Autodesk Inventor part; units mm, degrees
ref_plane "YZ Plane" through (0, 0, 0) normal (1, 0, 0) x (0, 1, 0)
ref_plane "XZ Plane" through (0, 0, 0) normal (0, 1, 0) x (-1, 0, 0)
ref_plane "XY Plane" through (0, 0, 0) normal (0, 0, 1) x (1, 0, 0)
ref_plane "Work Plane1" through (0, 0, 0) normal (0, 0, 1) x (1, 0, 0)
sketch "Sketch1" plane through (0, 0, 0) normal (0, 0, 1) x (1, 0, 0)
  circle A0 centre (-10, -25) radius 1.45
  circle A1 centre (-10, 25) radius 1.45
  circle A2 centre (10, 25) radius 1.45
  circle A3 centre (10, -25) radius 1.45
  circle A4 centre (-25, 25) radius 2.325
  circle A5 centre (25, -25) radius 2.325
  circle A6 centre (-25, -25) radius 2.325
  circle A7 centre (25, 25) radius 2.325
  line L0 (28, 30) -> (30, 28)
  line L1 (28, 30) -> (-28, 30)
  line L2 (-30, 28) -> (-28, 30)
  line L3 (-30, 28) -> (-30, -28)
  line L4 (-28, -30) -> (-30, -28)
  line L5 (-28, -30) -> (28, -30)
  line L6 (30, -28) -> (28, -30)
  line L7 (30, -28) -> (30, 28)
  circle A8 centre (-17.5, -17.5) radius 1.95
  circle A9 centre (17.5, 17.5) radius 1.95
  circle A10 centre (17.5, -17.5) radius 1.95
  circle A11 centre (-17.5, 17.5) radius 1.95
  circle A12 centre (0, 0) radius 7.5
  circle A13 centre (-25.33, -75.26) radius 6.15
  circle A14 centre (25, -10) radius 1.45
  circle A15 centre (-25, -10) radius 1.45
  circle A16 centre (-25, 10) radius 1.45
  circle A17 centre (25, 10) radius 1.45
  point P0 (0, 0)
extrude "Extrusion1" add sketch "Sketch1" along normal blind 8 contours L0 L7 L6 L5 L4 L3 L2 L1
sketch "Sketch2" plane through (0, 0, 8) normal (0, 0, 1) x (1, 0, 0)
  circle A0 centre (0, 0) radius 7.5
  circle A1 centre (25, 10) radius 1.45
  circle A2 centre (-25, 10) radius 1.45
  circle A3 centre (-25, -10) radius 1.45
  circle A4 centre (25, -10) radius 1.45
  circle A5 centre (10, -25) radius 1.45
  circle A6 centre (10, 25) radius 1.45
  circle A7 centre (-10, 25) radius 1.45
  circle A8 centre (-10, -25) radius 1.45
  line L0 (-28, -30) -> (28, -30)
  line L1 (28, -30) -> (30, -28)
  line L2 (30, -28) -> (30, 28)
  line L3 (30, 28) -> (28, 30)
  line L4 (28, 30) -> (-28, 30)
  line L5 (30, -28) -> (30, 28)
  line L6 (30, -30) -> (18, -30)
  line L7 (18, -30) -> (18, -80)
  line L8 (18, -80) -> (30, -80)
  line L9 (30, -80) -> (30, -30)
  line L10 (30, 28) -> (30, -28)
  line L11 (30, -30) -> (30, -28)
  line L12 (30, -28) -> (28, -30)
  line L13 (-28, 30) -> (-30, 28)
  line L14 (-30, 28) -> (-30, -28)
  line L15 (-30, -28) -> (-28, -30)
  line L16 (-30, -30) -> (-18, -30)
  line L17 (-18, -30) -> (-18, -80)
  line L18 (-18, -80) -> (-30, -80)
  line L19 (-30, -80) -> (-30, -30)
  line L20 (-30, -30) -> (-30, -28)
  line L21 (-30, -28) -> (-28, -30)
  line L22 (-28, -30) -> (-30, -30)
  line L23 (28, -30) -> (30, -28)
  line L24 (28, -30) -> (30, -30)
  line L25 (30, -30) -> (30, -28)
  line L26 (30, -28) -> (28, -30)
  circle A9 centre (-17.5, 17.5) radius 1.95
  circle A10 centre (-25, 25) radius 2.325
  circle A11 centre (25, 25) radius 2.325
  circle A12 centre (17.5, 17.5) radius 1.95
  circle A13 centre (17.5, -17.5) radius 1.95
  circle A14 centre (25, -25) radius 2.325
  circle A15 centre (-25, -25) radius 2.325
  point P0 (0, 0)
  point P1 (-24.2387, -104)
  dimension "d57" = 12
  dimension "d58" = 50
  dimension "d59" = 12
extrude "Extrusion2" add sketch "Sketch2" along normal blind 7
fillet "Fillet1" radius 4 6 edges at (30, -80, 11.5) (18, -80, 11.5) (-18, -80, 11.5) (-30, -80, 11.5) (-18, -30, 11.5) (18, -30, 11.5)
sketch "Sketch6" plane through (0, 0, 15) normal (0, 0, 1) x (1, 0, 0)
  line L0 (30, -76) -> (30, 28)
  line L1 (30, 28) -> (28, 30)
  line L2 (28, 30) -> (-28, 30)
  circle A0 centre (-1.1442, -37.6316) radius 2.45
  circle A1 centre (-1.1442, -37.6316) radius 1.45 construction
  line L3 (-14, -30) -> (14, -30)
  line L4 (18, -34) -> (18, -76)
  line L5 (22, -80) -> (26, -80)
  line L6 (-28, 30) -> (-30, 28)
  line L7 (-30, 28) -> (-30, -76)
  line L8 (-26, -80) -> (-22, -80)
  line L9 (-18, -76) -> (-18, -34)
  arc A2 (-30, -76) -> (-26, -80) centre (-26, -76) ccw
  arc A3 (-22, -80) -> (-18, -76) centre (-22, -76) ccw
  arc A4 (-14, -30) -> (-18, -34) centre (-14, -34) ccw
  arc A5 (18, -34) -> (14, -30) centre (14, -34) ccw
  arc A6 (18, -76) -> (22, -80) centre (22, -76) ccw
  arc A7 (26, -80) -> (30, -76) centre (26, -76) ccw
  point P0 (0, 0)
  dimension "d27" = 4.9
extrude "Extrusion6" cut sketch "Sketch6" against normal blind 4 contours A0
ref_plane "Work Plane2" through (-6, -91, 19) normal (1, 0, 0) x (0, 0, -1)
sketch "Sketch7" plane through (0, 0, 15) normal (0, 0, 1) x (1, 0, 0)
  circle A0 centre (10, -25) radius 1.45
  circle A1 centre (-10, -25) radius 1.45
  circle A2 centre (-25, -10) radius 1.45
  circle A3 centre (-25, 10) radius 1.45
  circle A4 centre (-10, 25) radius 1.45
  circle A5 centre (10, 25) radius 1.45
  circle A6 centre (25, 10) radius 1.45
  circle A7 centre (25, -10) radius 1.45
  circle A8 centre (-25, 25) radius 2.325
  circle A9 centre (25, 25) radius 2.325
  circle A10 centre (25, -25) radius 2.325
  circle A11 centre (-25, -25) radius 2.325
  point P0 (0, 0)
hole "Hole1" at (-25, -10, 15) at (-25, 10, 15) at (-10, 25, 15) at (10, 25, 15) at (25, 10, 15) at (25, -10, 15) at (10, -25, 15) at (-10, -25, 15) at (-25, 25, 15) at (-25, -25, 15) at (25, -25, 15) at (25, 25, 15) direction (0, 0, -1) diameter 3.2 end through all counterbore diameter 8 counterbore depth 10
sketch "Sketch8" plane through (0, 0, 15) normal (0, 0, 1) x (1, 0, 0)
  circle A0 centre (0, 0) radius 16
  dimension "d41" = 32
extrude "Extrusion7" cut sketch "Sketch8" against normal through all
chamfer "Chamfer3" distance 5 angle 45 2 edges at (21, -30, 8) (-21, -30, 8)
sketch "Sketch10" plane through (0, 0, 8) normal (0, 0, -1) x (-1, 0, 0)
  line L0 (-23, -35) -> (-30, -28)
  line L1 (-30, -76) -> (-30, -28)
  arc A0 (-30, -76) -> (-26, -80) centre (-26, -76) ccw
  line L2 (-22, -80) -> (-26, -80)
  arc A1 (-22, -80) -> (-18, -76) centre (-22, -76) ccw
  line L3 (-18, -35) -> (-18, -76)
  line L4 (-23, -35) -> (-18, -35)
  line L5 (18, -35) -> (23, -35)
  line L6 (18, -35) -> (18, -76)
  arc A2 (18, -76) -> (22, -80) centre (22, -76) ccw
  line L7 (22, -80) -> (26, -80)
  arc A3 (26, -80) -> (30, -76) centre (26, -76) ccw
  line L8 (30, -28) -> (30, -76)
  line L9 (30, -28) -> (23, -35)
  circle A4 centre (-24, -70) radius 2.45
  circle A5 centre (24, -70) radius 2.45
  circle A6 centre (-24, -58) radius 2.45
  circle A7 centre (24, -58) radius 2.45
  circle A8 centre (-24, -46) radius 2.45
  circle A9 centre (24, -46) radius 2.45
  point P0 (0, 0)
  dimension "d63" = 4.9
  dimension "d64" = 4.9
  dimension "d65" = 4.9
  dimension "d66" = 4.9
  dimension "d67" = 4.9
  dimension "d68" = 4.9
  dimension "d69" = 10
  dimension "d70" = 12
  dimension "d71" = 12
  dimension "d72" = 10
  dimension "d73" = 12
  dimension "d74" = 12
extrude "Extrusion9" cut sketch "Sketch10" against normal blind 6 contours A4 | A5 | A6 | A7 | A8 | A9
properties part number "cellSTORM_UC2_Sample_arm"
Build history of the part. All positions in model axes, mm. A direction names the side the tool comes from. Coordinates: 2 decimals unless noted, no trailing zeros. Order: outer loops, then holes, each group sorted by start corner. A loop starts at its lowest first (then second) coordinate and runs counter-clockwise, first axis right, second up.
Item 1: Saw through at A-A on x = -10. List the corners of the cut face in (y, z), then the cut area to 3 significant figures.
Filled in:
outline: (-30, 0) - (-26.6, 0) - (-26.6, 5) - (-29, 5) - (-29, 15) - (-30, 15) - close; (-23.4, 0) - (-12.49, 0) - (-12.49, 15) - (-21, 15) - (-21, 5) - (-23.4, 5) - close; (12.49, 0) - (23.4, 0) - (23.4, 5) - (21, 5) - (21, 15) - (12.49, 15) - close; (26.6, 0) - (30, 0) - (30, 15) - (29, 15) - (29, 5) - (26.6, 5) - close
area: 333 mm2
Item 2: Saw through at D-D on y = -46. List the corners of the cut face in (x, z).
Filled in:
outline: (-30, 8) - (-26.45, 8) - (-26.45, 14) - (-21.55, 14) - (-21.55, 8) - (-18, 8) - (-18, 15) - (-30, 15) - close; (18, 8) - (21.55, 8) - (21.55, 14) - (26.45, 14) - (26.45, 8) - (30, 8) - (30, 15) - (18, 15) - close
Item 3: Drop flat-ended pins along their axis: pin 1 Ø1.2 at (x, y) = (-17, -18) entering from -Z; pin 2 Ø2.5 at (x, y) = (-8, -25.5) entering from +Z; pin 3 Ø4 at (x, y) = (24, -70) entering from -Z; pin 4 Ø6 at (x, y) = (-21, -11) entering from -Z. Give the stop position or say it passes through.
Filled in:
pin 1: stops at z = 8
pin 2: stops at z = 5
pin 3: stops at z = 14
pin 4: stops at z = 0
Item 4: Drill centre lines: L1, parallel to X at y = -25, z = 2.7 (3 decimals); L2, parallel to X at y = -10, z = 2.7; L3, parallel to X at y = -47, z = 13.5. Where is each one in solid material? Low to high.
Filled in:
L1: x = -30 to -27.325, -22.675 to -11.6, -8.4 to 8.4, 11.6 to 22.675, 27.325 to 30
L2: x = -30 to -26.6, -23.4 to -12.49, 12.49 to 23.4, 26.6 to 30
L3: x = -30 to -26.24, -21.76 to -18, 18 to 21.76, 26.24 to 30
Item 5: Saw through at B-B on z = 1.5. State how many separate pieces and enclosed holes the cut face has, then the cut area to 3 significant figures.
Filled in:
separate pieces: 1
enclosed holes: 17
area: 2,610 mm2
Item 6: Mould opens along X. For faces 4 (the flat face through (28, -30, 5)), 5 (the flat face through (24, -54, 8)), 6 (the flat face through (-24, -46, 14)), 7 (the flat face through (-10, 23, 5)) say: released by +X, released by -X, zero draft, split by the parting line, or undercut.
Filled in:
face 4: released by +X
face 5: zero draft
face 6: undercut
face 7: undercut
Item 7: Tool access for faces 1 (the cylindrical face through (12.4, 28.2, 9.9)), 2 (the flat face through (24, -46, 14)), 3 (the cylindrical face through (19.141, -78.797, 11.549)): list every direction of +Z, -Z, +X, -X, +Y, -Y with a clear straight run to the whole face (end or side of a thin tool).
Filled in:
face 1: +Z
face 2: -Z
face 3: +Z, -Z, -Y
